The listing builds one solid part. Answer for the finished solid, in the listing's coordinates (mm). Give positions to 0.01 mm unless a question says otherwise; leave off trailing zeros. Use a Markdown table: item, result. Add a question column.
1) A flat-ended cylindrical pin translates along its axis: pin 1 (0.8 mm diameter, centred on y = 25, z = 1, fed in from +X). Find the tip coordinate at first contact, or state that the pin passes through.
2) Find section A-A, the plane z = 0.7. State how many separate pieces and enclosed holes the cut face has, plus the area to 3 significant figures.
3) Straight lines are drawn through the part: line 1 (X direction, y = -5, z = 0.8); line 2 (Y direction, x = 1.5, z = 0.3); line 3 (X direction, y = 1, z = 1.1). For each, find the intervals that lie inside material, in ascending order.
from build123d import *

# Parameters (mm, degrees)
SKETCH_3_R      = 0.4499991
SKETCH_3_R_2    = 0.3999992
SKETCH_3_R_3    = 0.499999
EXTRUDE_1_DEPTH = 1.5


with BuildPart() as part:
    # Эскиз3 → Бобышка-Вытянуть1 (new body)
    with BuildSketch(Plane.XY):
        Polygon((24.081237265, -17.758826004), (24.081237265, 22.241173056), (19.081237265, 22.241173056), (19.081237265, 27.241173056), (-20.918761795, 27.241173056), (-20.918761795, 22.241173056), (-25.918761795, 22.241173056), (-25.918761795, -17.758826004), (-20.918761795, -17.758826004), (-20.918761795, -22.758826004), (19.081237265, -22.758826004), (19.081237265, -17.758826004), align=None)
        with Locations((22.581258045, 1.241166636)):
            Circle(SKETCH_3_R, mode=Mode.SUBTRACT)
        with Locations((22.581258045, 3.791174236)):
            Circle(SKETCH_3_R, mode=Mode.SUBTRACT)
        with Locations((22.581258045, 6.341181836)):
            Circle(SKETCH_3_R, mode=Mode.SUBTRACT)
        with Locations((22.581258045, 8.891189436)):
            Circle(SKETCH_3_R, mode=Mode.SUBTRACT)
        with Locations((22.581258045, 11.441197036)):
            Circle(SKETCH_3_R, mode=Mode.SUBTRACT)
        with Locations((22.581258045, 13.991204636)):
            Circle(SKETCH_3_R, mode=Mode.SUBTRACT)
        with Locations((17.501258045, 3.791174236)):
            Circle(SKETCH_3_R, mode=Mode.SUBTRACT)
        with Locations((17.501258045, 6.341181836)):
            Circle(SKETCH_3_R, mode=Mode.SUBTRACT)
        with Locations((17.501258045, 8.891189436)):
            Circle(SKETCH_3_R, mode=Mode.SUBTRACT)
        with Locations((17.501258045, 11.441197036)):
            Circle(SKETCH_3_R, mode=Mode.SUBTRACT)
        with Locations((17.501258045, 13.991204636)):
            Circle(SKETCH_3_R, mode=Mode.SUBTRACT)
        with Locations((17.501258045, 16.541212236)):
            Circle(SKETCH_3_R, mode=Mode.SUBTRACT)
        with Locations((20.041258045, 16.541212236)):
            Circle(SKETCH_3_R, mode=Mode.SUBTRACT)
        with Locations((20.041258045, 13.991204636)):
            Circle(SKETCH_3_R, mode=Mode.SUBTRACT)
        with Locations((20.041258045, 11.441197036)):
            Circle(SKETCH_3_R, mode=Mode.SUBTRACT)
        with Locations((20.041258045, 8.891189436)):
            Circle(SKETCH_3_R, mode=Mode.SUBTRACT)
        with Locations((20.041258045, 6.341181836)):
            Circle(SKETCH_3_R, mode=Mode.SUBTRACT)
        with Locations((20.041258045, 3.791174236)):
            Circle(SKETCH_3_R, mode=Mode.SUBTRACT)
        with Locations((20.041258045, 1.241166636)):
            Circle(SKETCH_3_R, mode=Mode.SUBTRACT)
        with Locations((22.581235185, -6.388825724)):
            Circle(SKETCH_3_R, mode=Mode.SUBTRACT)
        with Locations((22.581235185, -3.848825724)):
            Circle(SKETCH_3_R, mode=Mode.SUBTRACT)
        with Locations((22.581235185, -1.308825724)):
            Circle(SKETCH_3_R, mode=Mode.SUBTRACT)
        with Locations((3.011236225, 25.741170976)):
            Circle(SKETCH_3_R, mode=Mode.SUBTRACT)
        with Locations((5.551236225, 23.201170976)):
            Circle(SKETCH_3_R, mode=Mode.SUBTRACT)
        with Locations((5.551236225, 25.741170976)):
            Circle(SKETCH_3_R, mode=Mode.SUBTRACT)
        with Locations((8.091236225, 23.201170976)):
            Circle(SKETCH_3_R, mode=Mode.SUBTRACT)
        with Locations((8.091236225, 25.741170976)):
            Circle(SKETCH_3_R, mode=Mode.SUBTRACT)
        with Locations((10.631236225, 25.741170976)):
            Circle(SKETCH_3_R, mode=Mode.SUBTRACT)
        with Locations((10.631236225, 23.201170976)):
            Circle(SKETCH_3_R, mode=Mode.SUBTRACT)
        with Locations((13.706236425, 21.341172156)):
            Circle(SKETCH_3_R_2, mode=Mode.SUBTRACT)
        with Locations((15.206235965, 21.341172156)):
            Circle(SKETCH_3_R_2, mode=Mode.SUBTRACT)
        with Locations((16.706235505, 21.341172156)):
            Circle(SKETCH_3_R_2, mode=Mode.SUBTRACT)
        with Locations((6.656270845, 0.041156336)):
            Circle(SKETCH_3_R, mode=Mode.SUBTRACT)
        with Locations((6.656270845, -5.038843664)):
            Circle(SKETCH_3_R, mode=Mode.SUBTRACT)
        with Locations((6.656270845, -2.498843664)):
            Circle(SKETCH_3_R, mode=Mode.SUBTRACT)
        with Locations((9.131325585, -2.498843664)):
            Circle(SKETCH_3_R, mode=Mode.SUBTRACT)
        with Locations((9.131325585, -5.038843664)):
            Circle(SKETCH_3_R, mode=Mode.SUBTRACT)
        with Locations((11.681361125, -2.498843664)):
            Circle(SKETCH_3_R, mode=Mode.SUBTRACT)
        with Locations((14.261284845, -20.508802564)):
            Circle(SKETCH_3_R, mode=Mode.SUBTRACT)
        with Locations((11.721284845, -20.508802564)):
            Circle(SKETCH_3_R, mode=Mode.SUBTRACT)
        with Locations((9.181284845, -20.508802564)):
            Circle(SKETCH_3_R, mode=Mode.SUBTRACT)
        with Locations((1.598775245, -20.508802564)):
            Circle(SKETCH_3_R, mode=Mode.SUBTRACT)
        with Locations((-0.941224755, -20.508802564)):
            Circle(SKETCH_3_R, mode=Mode.SUBTRACT)
        with Locations((-3.481224755, -20.508802564)):
            Circle(SKETCH_3_R, mode=Mode.SUBTRACT)
        with Locations((-11.063734355, -20.508802564)):
            Circle(SKETCH_3_R, mode=Mode.SUBTRACT)
        with Locations((-13.603734355, -20.508802564)):
            Circle(SKETCH_3_R, mode=Mode.SUBTRACT)
        with Locations((-16.143734355, -20.508802564)):
            Circle(SKETCH_3_R, mode=Mode.SUBTRACT)
        with Locations((-22.668758135, 10.141171696)):
            Circle(SKETCH_3_R, mode=Mode.SUBTRACT)
        with Locations((-22.668758135, 12.681171696)):
            Circle(SKETCH_3_R, mode=Mode.SUBTRACT)
        with Locations((-7.333782455, 25.756172216)):
            Circle(SKETCH_3_R_3, mode=Mode.SUBTRACT)
        with Locations((-4.793782455, 25.756172216)):
            Circle(SKETCH_3_R_3, mode=Mode.SUBTRACT)
        with Locations((-2.253782455, 25.756172216)):
            Circle(SKETCH_3_R_3, mode=Mode.SUBTRACT)
        with Locations((0.286217545, 25.756172216)):
            Circle(SKETCH_3_R_3, mode=Mode.SUBTRACT)
        with Locations((3.011236225, 23.201170976)):
            Circle(SKETCH_3_R, mode=Mode.SUBTRACT)
        with Locations((11.681361125, -5.038843664)):
            Circle(SKETCH_3_R, mode=Mode.SUBTRACT)
        with Locations((-21.868764815, 17.476170996)):
            Circle(SKETCH_3_R, mode=Mode.SUBTRACT)
        with Locations((-21.868764815, 20.016170996)):
            Circle(SKETCH_3_R, mode=Mode.SUBTRACT)
        with Locations((-16.143764835, 23.341173236)):
            Circle(SKETCH_3_R, mode=Mode.SUBTRACT)
        with Locations((-13.603764835, 23.341173236)):
            Circle(SKETCH_3_R, mode=Mode.SUBTRACT)
    extrude(amount=EXTRUDE_1_DEPTH)


solid = part.part
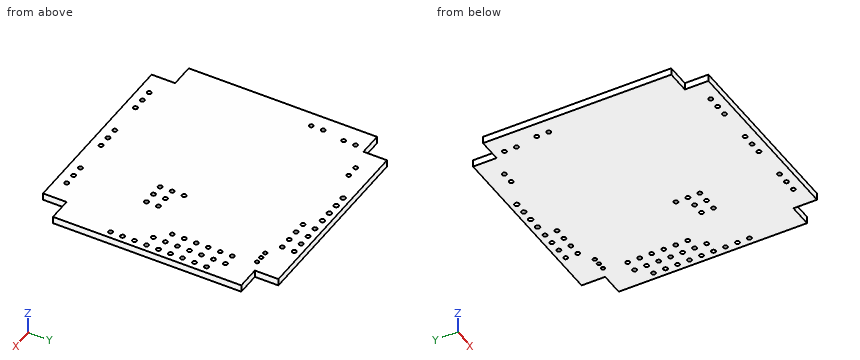
The answers:
| question | item | result |
|---|---|---|
| 1 | pin 1 | x = 19.08 |
| 2 | separate pieces | 1 |
| 2 | enclosed holes | 59 |
| 2 | area | 2,360 mm2 |
| 3 | line 1 | -25.92 to 6.21, 7.1 to 8.68, 9.58 to 11.23, 12.13 to 24.08 |
| 3 | line 2 | -22.76 to -20.95, -20.07 to 27.24 |
| 3 | line 3 | -25.92 to 19.66, 20.42 to 22.2, 22.96 to 24.08 |
